```python
from build123d import *

# Parameters (mm, degrees)
SKETCH2_W          = 6.32
SKETCH2_H          = 6.32
CUT_EXTRUDE1_DEPTH = 29
SKETCH3_R          = 0.5
CUT_EXTRUDE2_DEPTH = 6.5


with BuildPart() as part:
    # Sketch1 → Revolve1 (revolve)
    with BuildSketch(Plane.XY):
        Polygon((-9.5, 5.5), (9.5, 5.5), (9.5, 5), (14, 5), (14, 0), (-14, 0), (-14, 5), (-9.5, 5), align=None)
    revolve(axis=Axis((0, 0, 0), (-1, 0, 0)))

    # Sketch2 → Cut-Extrude1 (cut, through all)
    with BuildSketch(Plane.ZY.offset(14)):
        Rectangle(SKETCH2_W, SKETCH2_H)
    extrude(amount=-CUT_EXTRUDE1_DEPTH, mode=Mode.SUBTRACT)

    # Sketch3 → Cut-Extrude2 (cut, through all)
    with BuildSketch(Plane(origin=(0, 0, 0), x_dir=(1, 0, 0), z_dir=(0, 1, 0))):
        Circle(SKETCH3_R)
    extrude(amount=CUT_EXTRUDE2_DEPTH, mode=Mode.SUBTRACT)


solid = part.part
```
Input: part model. Units: mm. Frame: model coordinates. A direction names the side the tool comes from. Round coordinates to 2 decimals unless told otherwise and drop trailing zeros. Order: outer loops, then holes, each group sorted by start corner. A loop starts at its lowest first (then second) coordinate and runs counter-clockwise, first axis right, second up. Notation, with made-up numbers: (-24.75, 83) - (4.25, 83) arc R26 cw to (4.25, 115) - close; hole circle Ø4 at (60, 67.25). An arc over 180 degrees is marked (long way). One line per question, with ' | ' between items. Start each with the question number.
1) Cut plane D-D, the plane z = 0. Return the cut outline in (x, y).
2) Cut plane B-B, the plane z = -2. Return the cut outline in (x, y), then the cut area to 3 significant figures.
3) Cut plane A-A, the plane y = 0. Return the cut outline in (x, z).
4) Contact query for flat-ended pins moving along their axis: P1, Ø5, axis at x = 9.5, z = -2.5, coming from the -Y side; P2, Ø5, axis at x = 11, y = -4, coming from the -Z side; P3, Ø1, axis at x = -3, y = -4, coming from the +Z side. Output: stop coordinate, or through.
5) Ray query, probe 1 along Z at (x, y) = (4, 0); probe 2 along X at (y, z) = (4.85, 0); probe 3 along Z at (x, y) = (-13, 0). Return the intervals inside material, ascending.
6) Cut plane C-C, the plane x = -4.5. Return the cut outline in (y, z), then the cut area to 3 significant figures.
7) Pull-direction query (Y, two-part tool) for faces 4 (the flat face through (0, 0, 3.16)), 5 (the flat face through (0, 3.16, -1)), 6 (the flat face through (9.5, 1.6, 4.9)), 7 (the cylindrical face through (0.13, -1.19, 5.37)); classes: +Y half, -Y half, draft (parallel to the pull), parting line (faces both ways), or undercut.
8) Set-up query: faces 1 (the cylindrical face through (0.231, 4.314, 0.444)), 2 (the cylindrical face through (11.78, -1.08, 4.88)), 3 (the flat face through (-9.5, -1.6, 4.9)). Return all of +Z, -Z, +X, -X, +Y, -Y with unobstructed straight access to the full face (end or side cutting, diameter ignored); none if empty.
Worked out:
1) outline: (-14, -5) - (-9.5, -5) - (-9.5, -5.5) - (9.5, -5.5) - (9.5, -5) - (14, -5) - (14, -3.16) - (-14, -3.16) - close; (-14, 3.16) - (-0.5, 3.16) - (-0.5, 5.5) - (-9.5, 5.5) - (-9.5, 5) - (-14, 5) - close; (0.5, 3.16) - (14, 3.16) - (14, 5) - (9.5, 5) - (9.5, 5.5) - (0.5, 5.5) - close
2) outline: (-14, -4.58) - (-9.5, -4.58) - (-9.5, -5.12) - (9.5, -5.12) - (9.5, -4.58) - (14, -4.58) - (14, -3.16) - (-14, -3.16) - close; (-14, 3.16) - (14, 3.16) - (14, 4.58) - (9.5, 4.58) - (9.5, 5.12) - (-9.5, 5.12) - (-9.5, 4.58) - (-14, 4.58) - close | area: 100 mm^2
3) outline: (-14, -5) - (-9.5, -5) - (-9.5, -5.5) - (9.5, -5.5) - (9.5, -5) - (14, -5) - (14, -3.16) - (-14, -3.16) - close; (-14, 3.16) - (14, 3.16) - (14, 5) - (9.5, 5) - (9.5, 5.5) - (-9.5, 5.5) - (-9.5, 5) - (-14, 5) - close
4) P1: stops at y = -5.5 | P2: stops at z = -5.12 | P3: stops at z = 4.24
5) probe 1: z = -5.5 to -3.16, 3.16 to 5.5 | probe 2: x = -14 to -0.5, 0.5 to 14 | probe 3: z = -5 to -3.16, 3.16 to 5
6) outline: circle Ø11 at (0, 0); hole (-3.16, -3.16) - (3.16, -3.16) - (3.16, 3.16) - (-3.16, 3.16) - close | area: 55.1 mm^2
7) face 4: undercut | face 5: undercut | face 6: draft | face 7: parting line
8) face 1: +Y | face 2: +X | face 3: -X
